Geometry: final body of the model. Coordinates: model frame, mm. Face numbers are marked on the shaded views. A direction names the side the tool comes from. Give positions to 0.01 mm unless a question says otherwise; leave off trailing zeros. Loops run counter-clockwise (first coordinate to the right, second up) from the corner with the lowest first, then second, coordinate; pieces in that order, holes last.
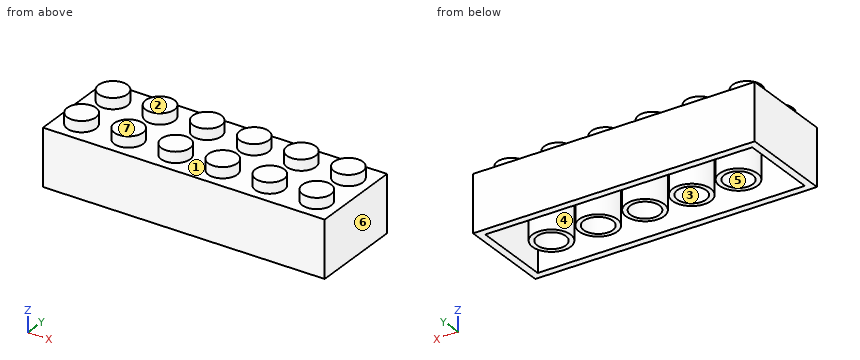
from build123d import *

# Parameters (mm, degrees)
F0_W      = 47.752
F0_H      = 15.8242
F0_R      = 2.4511
F1_DEPTH  = 9.6012
F2_DEPTH  = 11.43
F3_W      = 45.2628
F3_H      = 13.335
F3_R      = 3.2258
F4_DEPTH  = 7.62
F5_DEPTH  = 8.2804
F6_R      = 2.413
F7_DEPTH  = 7.62
F8_R      = 2.448528
F9_DEPTH  = 7.62
F10_R     = 2.453665
F11_DEPTH = 7.62
F12_R     = 2.460778
F13_DEPTH = 7.62
F14_R     = 2.432701
F15_DEPTH = 7.62


with BuildPart() as f1:
    # F0 (on Top) → F1 (new body)
    with BuildSketch(Plane.XY):
        Rectangle(F0_W, F0_H)
        with Locations((-19.9517, -3.9878)):
            Circle(F0_R, mode=Mode.SUBTRACT)
        with Locations((-11.9761, -3.9878)):
            Circle(F0_R, mode=Mode.SUBTRACT)
        with Locations((-4.0005, -3.9878)):
            Circle(F0_R, mode=Mode.SUBTRACT)
        with Locations((3.9751, -3.9878)):
            Circle(F0_R, mode=Mode.SUBTRACT)
        with Locations((11.9507, -3.9878)):
            Circle(F0_R, mode=Mode.SUBTRACT)
        with Locations((19.9263, -3.9878)):
            Circle(F0_R, mode=Mode.SUBTRACT)
        with Locations((-19.9517, 3.9878)):
            Circle(F0_R, mode=Mode.SUBTRACT)
        with Locations((-11.97102, 3.9878)):
            Circle(F0_R, mode=Mode.SUBTRACT)
        with Locations((-3.99034, 3.9878)):
            Circle(F0_R, mode=Mode.SUBTRACT)
        with Locations((3.99034, 3.9878)):
            Circle(F0_R, mode=Mode.SUBTRACT)
        with Locations((11.97102, 3.9878)):
            Circle(F0_R, mode=Mode.SUBTRACT)
        with Locations((19.9517, 3.9878)):
            Circle(F0_R, mode=Mode.SUBTRACT)
        with Locations((-19.9517, 3.9878)):
            Circle(F0_R)
        with Locations((-19.9517, -3.9878)):
            Circle(F0_R)
        with Locations((-11.9761, -3.9878)):
            Circle(F0_R)
        with Locations((-11.97102, 3.9878)):
            Circle(F0_R)
        with Locations((-3.99034, 3.9878)):
            Circle(F0_R)
        with Locations((-4.0005, -3.9878)):
            Circle(F0_R)
        with Locations((3.9751, -3.9878)):
            Circle(F0_R)
        with Locations((3.99034, 3.9878)):
            Circle(F0_R)
        with Locations((11.9507, -3.9878)):
            Circle(F0_R)
        with Locations((11.97102, 3.9878)):
            Circle(F0_R)
        with Locations((19.9263, -3.9878)):
            Circle(F0_R)
        with Locations((19.9517, 3.9878)):
            Circle(F0_R)
    extrude(amount=F1_DEPTH)

    # F0 (on Top) → F2 (join)
    with BuildSketch(Plane.XY):
        with Locations((-11.9761, -3.9878)):
            Circle(F0_R)
        with Locations((-19.9517, -3.9878)):
            Circle(F0_R)
        with Locations((-4.0005, -3.9878)):
            Circle(F0_R)
        with Locations((3.9751, -3.9878)):
            Circle(F0_R)
        with Locations((11.9507, -3.9878)):
            Circle(F0_R)
        with Locations((19.9263, -3.9878)):
            Circle(F0_R)
        with Locations((3.99034, 3.9878)):
            Circle(F0_R)
        with Locations((11.97102, 3.9878)):
            Circle(F0_R)
        with Locations((19.9517, 3.9878)):
            Circle(F0_R)
        with Locations((-3.99034, 3.9878)):
            Circle(F0_R)
        with Locations((-11.97102, 3.9878)):
            Circle(F0_R)
        with Locations((-19.9517, 3.9878)):
            Circle(F0_R)
    extrude(amount=F2_DEPTH)

    # F3 (on face) → F4 (join)
    with BuildSketch(Plane(origin=(0, 0, 0), x_dir=(1, 0, 0), z_dir=(0, 0, -1))):
        Rectangle(F3_W, F3_H)
        with Locations((-15.8496, 0)):
            Circle(F3_R, mode=Mode.SUBTRACT)
        with Locations((-7.9248, 0)):
            Circle(F3_R, mode=Mode.SUBTRACT)
        Circle(F3_R, mode=Mode.SUBTRACT)
        with Locations((7.9248, 0)):
            Circle(F3_R, mode=Mode.SUBTRACT)
        with Locations((15.8496, 0)):
            Circle(F3_R, mode=Mode.SUBTRACT)
    extrude(amount=-F4_DEPTH)

    # F3 (on face) → F5 (cut)
    with BuildSketch(Plane(origin=(0, 0, 0), x_dir=(1, 0, 0), z_dir=(0, 0, -1))):
        Rectangle(F3_W, F3_H)
        with Locations((-15.8496, 0)):
            Circle(F3_R, mode=Mode.SUBTRACT)
        with Locations((-7.9248, 0)):
            Circle(F3_R, mode=Mode.SUBTRACT)
        Circle(F3_R, mode=Mode.SUBTRACT)
        with Locations((7.9248, 0)):
            Circle(F3_R, mode=Mode.SUBTRACT)
        with Locations((15.8496, 0)):
            Circle(F3_R, mode=Mode.SUBTRACT)
    extrude(amount=-F5_DEPTH, mode=Mode.SUBTRACT)

    # F6 (on face) → F7 (cut)
    with BuildSketch(Plane(origin=(0, 0, 0), x_dir=(1, 0, 0), z_dir=(0, 0, -1))):
        with Locations((-15.8496, 0)):
            Circle(F6_R)
    extrude(amount=-F7_DEPTH, mode=Mode.SUBTRACT)

    # F8 (on face) → F9 (cut)
    with BuildSketch(Plane(origin=(0, 0, 0), x_dir=(1, 0, 0), z_dir=(0, 0, -1))):
        with Locations((-7.9248, 0)):
            Circle(F8_R)
    extrude(amount=-F9_DEPTH, mode=Mode.SUBTRACT)

    # F10 (on face) → F11 (cut)
    with BuildSketch(Plane(origin=(0, 0, 0), x_dir=(1, 0, 0), z_dir=(0, 0, -1))):
        Circle(F10_R)
    extrude(amount=-F11_DEPTH, mode=Mode.SUBTRACT)

    # F12 (on face) → F13 (cut)
    with BuildSketch(Plane(origin=(0, 0, 0), x_dir=(1, 0, 0), z_dir=(0, 0, -1))):
        with Locations((7.9248, 0)):
            Circle(F12_R)
    extrude(amount=-F13_DEPTH, mode=Mode.SUBTRACT)

    # F14 (on face) → F15 (cut)
    with BuildSketch(Plane(origin=(0, 0, 0), x_dir=(1, 0, 0), z_dir=(0, 0, -1))):
        with Locations((15.8496, 0)):
            Circle(F14_R)
    extrude(amount=-F15_DEPTH, mode=Mode.SUBTRACT)


solid = f1.part
Item 1: Draft query along X for the marked faces 4, 5, 6 and 7. Return one class per face: +X half, -X half, draft (parallel to the pull), parting line (faces both ways), or undercut.
Values follow:
face 4: undercut
face 5: undercut
face 6: +X half
face 7: draft
Item 2: Set-up query: the marked faces 1, 2 and 3. Return all of +Z, -Z, +X, -X, +Y, -Y with unobstructed straight access to the full face (end or side cutting, diameter ignored); none if empty.
Values follow:
face 1: +Z
face 2: +Z, +X, -X, +Y, -Y
face 3: -Z
Item 3: Section query D-D on x = -9. Return loops of the section in (y, z), plus the area to 3 significant figures.
Values follow:
outline: (-7.91, 0) - (-6.67, 0) - (-6.67, 8.28) - (-3.04, 8.28) - (-3.04, 0) - (-2.2, 0) - (-2.2, 7.62) - (2.2, 7.62) - (2.2, 0) - (3.04, 0) - (3.04, 8.28) - (6.67, 8.28) - (6.67, 0) - (7.91, 0) - (7.91, 9.6) - (-7.91, 9.6) - close
area: 58.4 mm2
Item 4: Section query A-A on z = 5.5. Give the number of separate pieces and of enclosed holes in the cut face, plus the area to 3 significant figures.
Values follow:
separate pieces: 6
enclosed holes: 6
area: 222 mm2
Item 5: Section query B-B on x = 0. Return loops of the section in (y, z).
Values follow:
outline: (-7.91, 0) - (-6.67, 0) - (-6.67, 8.28) - (-3.23, 8.28) - (-3.23, 0) - (-2.45, 0) - (-2.45, 7.62) - (2.45, 7.62) - (2.45, 0) - (3.23, 0) - (3.23, 8.28) - (6.67, 8.28) - (6.67, 0) - (7.91, 0) - (7.91, 9.6) - (-7.91, 9.6) - close
Item 6: Pin query (flat end, axial travel): pin 1 (1.4 mm diameter, centred on x = -15.5, y = 0.5, fed in from -Z); pin 2 (4 mm diameter, centred on x = 15.85, y = 0, fed in from +Z). Return the tip coordinate at first contact, or that it passes through.
Values follow:
pin 1: stops at z = 7.62
pin 2: stops at z = 9.6
Item 7: Ray query, probe 1 along Y at (x, z) = (-21, 3.5); probe 2 along X at (y, z) = (6.25, 6.5); probe 3 along Y at (x, z) = (-9, 3.5). Return the intervals inside material, ascending.
Values follow:
probe 1: y = -7.91 to -6.67, 6.67 to 7.91
probe 2: x = -23.88 to -22.63, 22.63 to 23.88
probe 3: y = -7.91 to -6.67, -3.04 to -2.2, 2.2 to 3.04, 6.67 to 7.91
